from build123d import *

# Parameters (mm, degrees)
F0_W     = 32
F0_H     = 45
F0_R     = 3
F1_DEPTH = 7
F2_R     = 3


with BuildPart() as f1:
    # F0 (on Front) → F1 (new body)
    with BuildSketch(Plane.XZ):
        with Locations((16, 22.5)):
            Rectangle(F0_W, F0_H)
        with Locations((16, 30)):
            Circle(F0_R, mode=Mode.SUBTRACT)
    extrude(amount=F1_DEPTH)

    # F2
    f2_edges = [f1.edges().sort_by_distance(p)[0] for p in [
        (32, -3.5, 45),
        (0, -3.5, 45),
        (16, -7, 45),
    ]]
    fillet(f2_edges, radius=F2_R)


solid = f1.part
Source: CAD feature listing. Evaluate the final solid. Frame: model axes, mm. Give positions to 0.01 mm unless a question says otherwise; leave off trailing zeros. Order: outer loops, then holes, each group sorted by start corner. A loop starts at its lowest first (then second) coordinate and runs counter-clockwise, first axis right, second up. Notation, with made-up numbers: (-30.75, -13.5) -> (-25.75, -13.5) arc R20 cw to (-25.75, 7.5) -> close; hole circle Ø6 at (-7.5, -15). An arc over 180 degrees is marked (long way). Use a Markdown table: item, result.
1) Ray query, line 1 along Z through (x, y) = (16, -3.75); line 2 along Z through (x, y) = (15, -3.25); line 3 along Z through (x, y) = (28, -4.25). Return the intervals inside material, ascending. Write a range as [from, to].
Answer list:
| item | result |
|---|---|
| line 1 | [0, 27], [33, 45] |
| line 2 | [0, 27.17], [32.83, 45] |
| line 3 | [0, 44.99] |
2) Section query D-D, the plane y = -6.25. Return the cut outline in (x, z), then the cut area to 3 significant figures.
Answer list:
| item | result |
|---|---|
| outline | (0, 0) -> (32, 0) -> (32, 42) arc R3 ccw to (31.25, 43.98) -> (0.75, 43.98) arc R3 ccw to (0, 42) -> close; hole circle Ø6 at (16, 30) |
| area | 1,380 mm² |
3) Mould query, pull axis Z, two halves, no side actions, for faces 1 (the flat face through (16, 0, 23)), 2 (the cylindrical face through (13.79, -3.45, 32.03)), 3 (the flat face through (16, -3, 0)), 4 (the cylindrical face through (31.1, -2.77, 44.14)). Classes: +Z half, -Z half, draft (parallel to the pull), parting line (faces both ways), or undercut.
Answer list:
| item | result |
|---|---|
| face 1 | draft |
| face 2 | undercut |
| face 3 | -Z half |
| face 4 | +Z half |
4) Section query C-C, the plane y = -2.5. Return the cut outline in (x, z).
Answer list:
| item | result |
|---|---|
| outline | (0, 0) -> (32, 0) -> (32, 42) arc R3 ccw to (29, 45) -> (3, 45) arc R3 ccw to (0, 42) -> close; hole circle Ø6 at (16, 30) |
5) Section query B-B, the plane x = 16. Return the cut outline in (y, z).
Answer list:
| item | result |
|---|---|
| outline | (-7, 0) -> (0, 0) -> (0, 27) -> (-7, 27) -> close; (-7, 33) -> (0, 33) -> (0, 45) -> (-4, 45) arc R3 ccw to (-7, 42) -> close |
6) Section query A-A, the plane z = 30. Return the cut outline in (x, y).
Answer list:
| item | result |
|---|---|
| outline | (0, -7) -> (13, -7) -> (13, 0) -> (0, 0) -> close; (19, -7) -> (32, -7) -> (32, 0) -> (19, 0) -> close |
7) Contact query for a flat-ended pin moving along its axis: P1, Ø6, axis at x = 9.5, z = 24.5, coming from the +Y side. Output: stop coordinate, or through.
Answer list:
| item | result |
|---|---|
| P1 | y = 0 |
